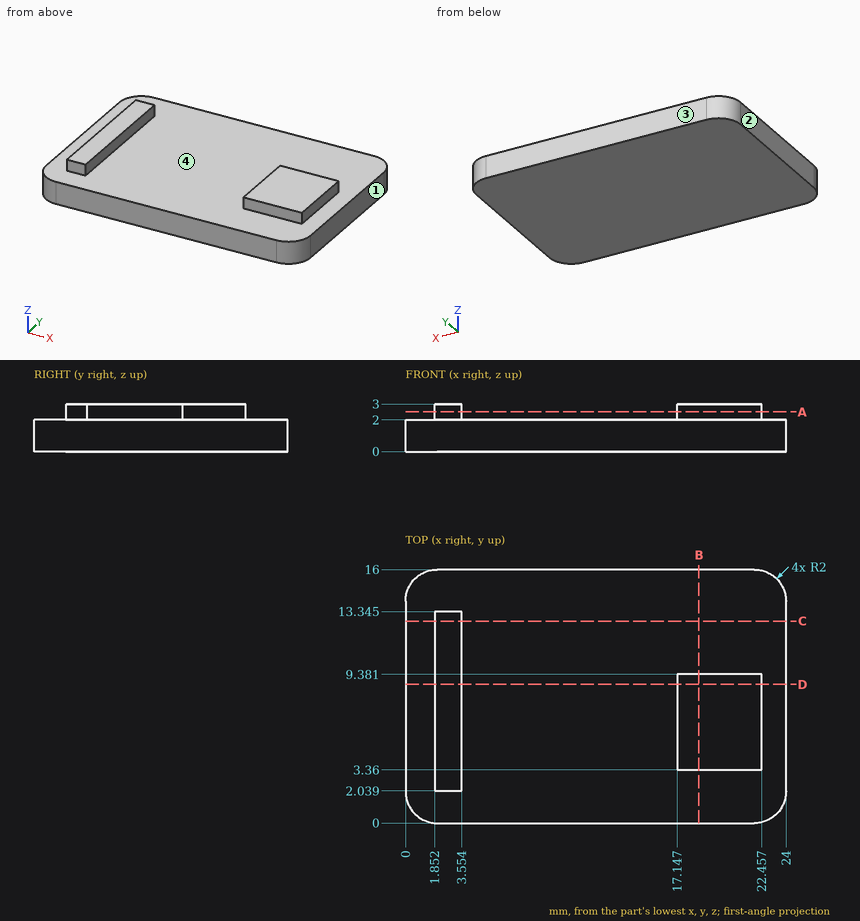
Check sheet for the drawn part. Datum: minimum x, y, z corner. Units: mm. Round coordinates to 2 decimals unless told otherwise and drop trailing zeros. Write each loop counter-clockwise with the first axis right and the second up, starting at its lowest first coordinate (ties: lowest second). Pieces come first, ordered by that corner, then holes. Notation, with made-up numbers: (3, -27) -> (8, -27) arc R33 ccw to (8, 3) -> close; hole circle Ø1 at (31, 56). An arc over 180 degrees is marked (long way). Write each question's results on one line, items separated by ' | '. Start each with the question number.
1. Material ranges on probe 1 along X at (y, z) = (6.5, 2.3); probe 2 along Z at (x, y) = (12, 10); probe 3 along Y at (x, z) = (17.75, 2.65), recorded low to high. Write a range as from..to.
2. Cross-section at C-C (y = 12.75). Enter the section's corners in (x, z).
3. Cross-section at A-A (z = 2.5). Enter the section's corners in (x, y) (1 decimal).
4. Cross-section at D-D (y = 8.75). Enter the section's corners in (x, z).
5. Cross-section at B-B (x = 18.5). Enter the section's corners in (y, z).
6. Draft check along X on the marked faces 1, 2, 3 and 4. Enter one of: +X half, -X half, draft (parallel to the pull), parting line (faces both ways), or undercut.
7. Depth check by flat-ended pin: P1, Ø0.8, axis at y = 7, z = 2.5, coming from the +X side; P2, Ø0.8, axis at x = 21, z = 2.5, coming from the +Y side; P3, Ø0.5, axis at x = 19.5, z = 2.5, coming from the -Y side. Enter the tip coordinate at first touch or a pass-through.
Solutions:
1) probe 1: x = 1.85..3.55, 17.15..22.46 | probe 2: z = 0..2 | probe 3: y = 3.36..9.38
2) outline: (0, 0) -> (24, 0) -> (24, 2) -> (3.55, 2) -> (3.55, 3) -> (1.85, 3) -> (1.85, 2) -> (0, 2) -> close
3) outline: (1.9, 2) -> (3.6, 2) -> (3.6, 13.3) -> (1.9, 13.3) -> close; (17.1, 3.4) -> (22.5, 3.4) -> (22.5, 9.4) -> (17.1, 9.4) -> close
4) outline: (0, 0) -> (24, 0) -> (24, 2) -> (22.46, 2) -> (22.46, 3) -> (17.15, 3) -> (17.15, 2) -> (3.55, 2) -> (3.55, 3) -> (1.85, 3) -> (1.85, 2) -> (0, 2) -> close
5) outline: (0, 0) -> (16, 0) -> (16, 2) -> (9.38, 2) -> (9.38, 3) -> (3.36, 3) -> (3.36, 2) -> (0, 2) -> close
6) face 1: +X half | face 2: -X half | face 3: draft | face 4: undercut
7) P1: stops at x = 22.46 | P2: stops at y = 9.38 | P3: stops at y = 3.36
